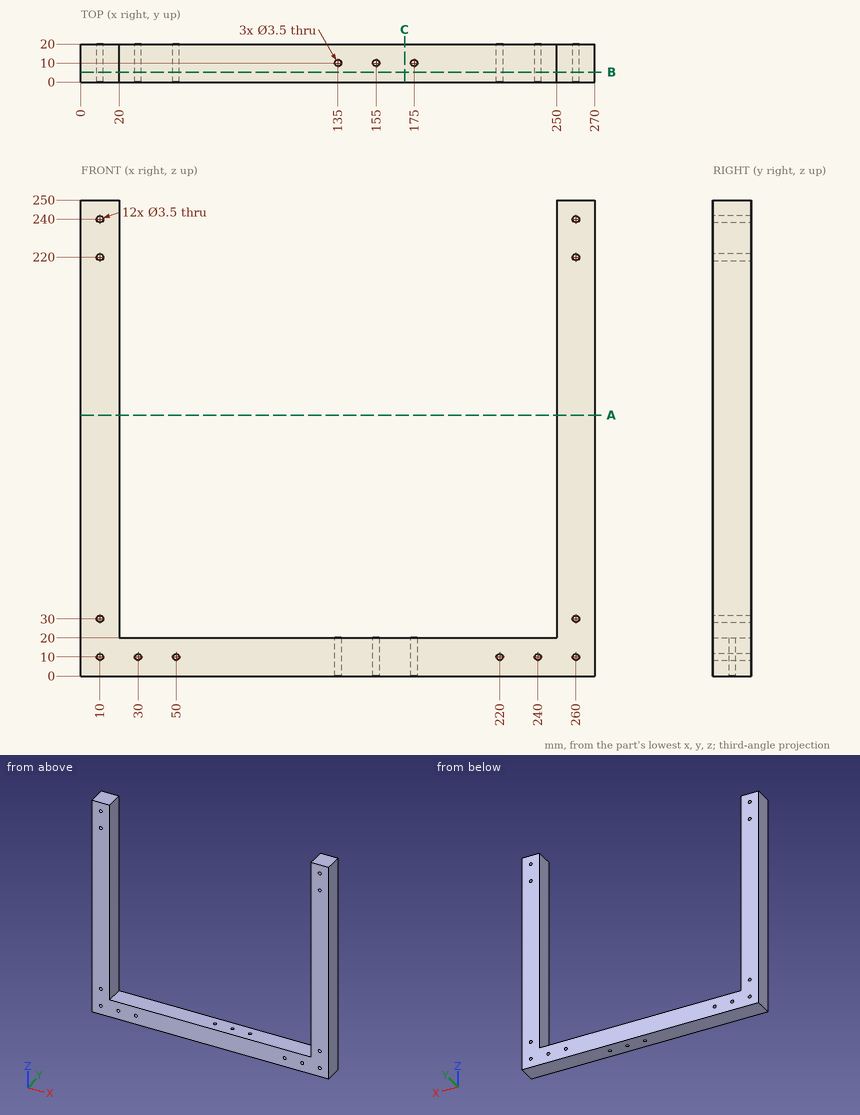
The figure shows three views and two pictorial views of one solid part (mm, origin at its lowest corner). Answer the questions. Coordinates: 2 decimals unless noted, no trailing zeros. Write each loop counter-clockwise with the first axis right and the second up, starting at its lowest first coordinate (ties: lowest second). Pieces come first, ordered by that corner, then holes. Notation, with made-up numbers: (19, -13.75) -> (61, -13.75) arc R17 cw to (61, -4.75) -> close; hole circle Ø8 at (38.25, 24.5). An arc over 180 degrees is marked (long way). Answer as a JSON object with one key per item and string values.
Q1. Consider line 1 (X direction, y = 13.75, z = 30); line 2 (Z direction, x = 260, y = 12.5); line 3 (Y direction, x = 155, z = 10.25). Determine where each line is inside the solid, lowest interval first. Write a range as [from, to].
The answers:
{"line 1": "x = [0, 8.25], [11.75, 20], [250, 258.25], [261.75, 270]", "line 2": "z = [0, 8.25], [11.75, 28.25], [31.75, 218.25], [221.75, 238.25], [241.75, 250]", "line 3": "y = [0, 8.25], [11.75, 20]"}
Q2. The part is cut by section A-A on z = 137. Give the vertices of the cut face in (x, y), then the cut area to 3 significant figures.
The answers:
{"outline": "(0, 0) -> (20, 0) -> (20, 20) -> (0, 20) -> close; (250, 0) -> (270, 0) -> (270, 20) -> (250, 20) -> close", "area": "800 mm2"}
Q3. The part is cut by section C-C on x = 170. Give the vertices of the cut face in (y, z), then the cut area to 3 significant figures.
The answers:
{"outline": "(0, 0) -> (20, 0) -> (20, 20) -> (0, 20) -> close", "area": "400 mm2"}
Q4. Flat-ended cylindrical pins translate along their axes: pin 1 Ø3 at (x, z) = (50, 10) entering from +Y (3 decimals); pin 2 Ø6 at (x, y) = (134.5, 10.5) entering from +Z. Find the tip coordinate at first contact, or state that the pin passes through.
The answers:
{"pin 1": "passes through", "pin 2": "stops at z = 20"}
Q5. The part is cut by section B-B on y = 5.25. Give the number of separate pieces and of enclosed holes in the cut face, then the cut area to 3 significant figures.
The answers:
{"separate pieces": "1", "enclosed holes": "12", "area": "14,500 mm2"}
